Can you work these out from the model? Positions are in its coordinate system, mm. A direction names the side the tool comes from. Round coordinates to 2 decimals unless told otherwise and drop trailing zeros. Order: outer loops, then holes, each group sorted by start corner. A loop starts at its lowest first (then second) coordinate and runs counter-clockwise, first axis right, second up.
from build123d import *

# Parameters (mm, degrees)
SKETCH1_W                                      = 12.7
SKETCH1_H                                      = 96.5962
EXTRUDE1_DEPTH                                 = 5.08
SKETCH2_W                                      = 12.7
SKETCH2_H                                      = 5.1562
EXTRUDE2_DEPTH                                 = 25.4
SKETCH6_W                                      = 12.7
SKETCH6_H                                      = 22.86
EXTRUDE4_DEPTH                                 = 7.62
F_4_CLEARANCE_HOLE1_D                          = 3.4544
SKETCH7_W                                      = 7.9248
SKETCH7_H                                      = 15.24
EXTRUDE5_DEPTH                                 = 3.175
FILLET1_R                                      = 1.27
FILLET2_R                                      = 6.35
CHAMFER1_SIZE                                  = 0.762
CBORE_FOR_4_SOCKET_HEAD_CAP_SCREW1_D           = 3.4544
CBORE_FOR_4_SOCKET_HEAD_CAP_SCREW1_CBORE_D     = 5.55752
CBORE_FOR_4_SOCKET_HEAD_CAP_SCREW1_CBORE_DEPTH = 2.8448


with BuildPart() as part:
    # Sketch1 → Extrude1 (new body)
    with BuildSketch(Plane.XY):
        with Locations((6.35, -48.2981)):
            Rectangle(SKETCH1_W, SKETCH1_H)
    extrude(amount=EXTRUDE1_DEPTH)

    # Sketch2 → Extrude2 (add)
    with BuildSketch(Plane(origin=(0, 0, 0), x_dir=(-1, 0, 0), z_dir=(0, 0, -1))):
        with Locations((-6.35, -2.5781)):
            Rectangle(SKETCH2_W, SKETCH2_H)
    extrude(amount=EXTRUDE2_DEPTH)

    # Sketch6 → Extrude4 (add)
    with BuildSketch(Plane(origin=(0, 0, 0), x_dir=(-1, 0, 0), z_dir=(0, 0, -1))):
        with Locations((-6.35, -85.1662)):
            Rectangle(SKETCH6_W, SKETCH6_H)
    extrude(amount=EXTRUDE4_DEPTH)

    # #4 Clearance Hole1 (through all)
    with Locations(Plane(origin=(0, 0, 0), x_dir=(-1, 0, 0), z_dir=(0, 1, 0))):
        with Locations((-8.89, -21.59), (-8.89, -13.97)):
            Hole(F_4_CLEARANCE_HOLE1_D / 2)

    # Sketch7 → Extrude5 (cut)
    with BuildSketch(Plane(origin=(0, 0, 0), x_dir=(1, 0, 0), z_dir=(0, 1, 0))):
        with Locations((8.7376, 17.78)):
            Rectangle(SKETCH7_W, SKETCH7_H)
    extrude(amount=-EXTRUDE5_DEPTH, mode=Mode.SUBTRACT)

    # Fillet1
    fillet1_edges = [part.edges().sort_by_distance(p)[0] for p in [
        (4.7752, -1.5875, -10.16),
    ]]
    fillet(fillet1_edges, radius=FILLET1_R)

    # Fillet2
    fillet2_edges = [part.edges().sort_by_distance(p)[0] for p in [
        (6.35, -73.7362, 0),
        (6.35, -5.1562, 0),
    ]]
    fillet(fillet2_edges, radius=FILLET2_R)

    # Chamfer1
    chamfer1_edges = [part.edges().sort_by_distance(p)[0] for p in [
        (12.7, -48.2981, 5.08),
        (6.35, 0, 5.08),
        (0, -48.2981, 5.08),
        (6.35, -96.5962, 5.08),
    ]]
    chamfer(chamfer1_edges, length=CHAMFER1_SIZE)

    # CBORE for #4 Socket Head Cap Screw1 (through all)
    with Locations(Plane.XY.offset(5.08)):
        with Locations((4.445, -84.963), (4.445, -77.0382)):
            CounterBoreHole(CBORE_FOR_4_SOCKET_HEAD_CAP_SCREW1_D / 2, CBORE_FOR_4_SOCKET_HEAD_CAP_SCREW1_CBORE_D / 2, CBORE_FOR_4_SOCKET_HEAD_CAP_SCREW1_CBORE_DEPTH)


solid = part.part
(1) If we mould it in two halves opening along Y, with no side actions, what happens to faces 6 (the face through (6.261, -71.925, -1.91)), 7 (the face through (5, 0, -7)), 8 (the face through (6.4, -85, -7.62))? For each: pulls with the +Y half, pulls with the -Y half, needs draft (parallel to the pull), parting line crosses it, or undercut.
(2) I want a section at D-D, the plane y = -48. List the corners of the cut face in (x, z) for me, plus the area to 3 significant figures.
(3) I want a section at C-C, the plane z = -4. List the corners of the cut face in (x, y) for me (3 decimals), plus the area to 3 significant figures.
(4) I want a section at B-B, the plane z = -13.97. List the corners of the cut face in (x, y) for me (3 decimals), plus the area to 3 significant figures.
(5) Please list where these lines run through material, in increasing order: probe 1 along Y at (x, z) = (3.25, -4.5); probe 2 along Y at (x, z) = (10.75, -7); probe 3 along Y at (x, z) = (6, -5).
(6) I'm going to push flat-ended pins straight in: pin 1 Ø3.5 at (x, y) = (10, -2) entering from -Z; pin 2 Ø6 at (x, y) = (3, -60) entering from -Z; pin 3 Ø5.5 at (x, z) = (8.89, -21.59) entering from -Y; pin 4 Ø3 at (x, y) = (4, -86) entering from +Z. Where does each tip first touch, or does it pass through?
(7) I want a section at A-A, the plane x = 8.89. List the corners of the cut face in (y, z) for me (3 decimals), plus the area to 3 significant figures.
(8) On a 3-axis mill with a long thin cutter (end or side, diameter ignored), from which of +Z, -Z, +X, -X, +Y, -Y can I reach the whole of each face in a straight line? I mean faces 1 (the face through (6, -96.596, -2)), 2 (the face through (6, -39, 0)), 3 (the face through (4.775, -2, -18)), 4 (the face through (3.843, -87.676, 3.678)), 5 (the face through (7.62, -4.18, -20.42)). Say none if no direction works.
Ans:
1. face 6: undercut
1. face 7: pulls with the +Y half
1. face 8: needs draft
2. outline: (0, 0) - (12.7, 0) - (12.7, 4.32) - (11.94, 5.08) - (0.76, 5.08) - (0, 4.32) - close
2. area: 63.9 mm2
3. outline: (0, -96.596) - (12.7, -96.596) - (12.7, -73.285) - (0, -73.285) - close; (0, -5.607) - (12.7, -5.607) - (12.7, 0) - (0, 0) - close; hole circle Ø3.454 at (4.445, -84.963); hole circle Ø3.454 at (4.445, -77.038)
3. area: 349 mm2
4. outline: (0, -5.156) - (7.163, -5.156) - (7.163, -3.175) - (4.775, -3.175) - (4.775, 0) - (0, 0) - close; (10.617, -5.156) - (12.7, -5.156) - (12.7, -3.175) - (10.617, -3.175) - close
4. area: 33.5 mm2
5. probe 1: y = -96.6 to -86.21, -83.72 to -78.29, -75.79 to -73.46, -5.43 to 0
5. probe 2: y = -96.6 to -73.74, -5.16 to 0
5. probe 3: y = -96.6 to -85.71, -84.21 to -77.79, -76.29 to -73.59, -5.3 to 0
6. pin 1: stops at z = -25.4
6. pin 2: stops at z = 0
6. pin 3: stops at y = -5.16
6. pin 4: stops at z = 2.24
7. outline: (-96.596, -7.62) - (-73.736, -7.62) - (-73.736, -6.35) arc R6.35 cw to (-67.386, 0) - (-11.506, 0) arc R6.35 cw to (-5.156, -6.35) - (-5.156, -12.243) - (-3.175, -12.243) - (-3.175, -10.16) - (0, -10.16) - (0, 4.318) - (-0.762, 5.08) - (-95.834, 5.08) - (-96.596, 4.318) - close; (-5.156, -25.4) - (-3.175, -25.4) - (-3.175, -23.317) - (-5.156, -23.317) - close; (-5.156, -19.863) - (-3.175, -19.863) - (-3.175, -15.697) - (-5.156, -15.697) - close
7. area: 751 mm2
8. face 1: +Z, -Z, +X, -X, -Y
8. face 2: -Z, +X, -X
8. face 3: -Z, +X, +Y
8. face 4: +Z
8. face 5: +Y, -Y
